Input: part model. Units: mm. Frame: model coordinates. Face numbers are marked on the shaded views. Coordinates: 2 decimals unless noted, no trailing zeros. Order: outer loops, then holes, each group sorted by start corner. A loop starts at its lowest first (then second) coordinate and runs counter-clockwise, first axis right, second up. Notation, with made-up numbers: (24.25, 63) - (73.25, 63) arc R32 cw to (73.25, 99) - close; hole circle Ø7 at (41, -28.5). An arc over 180 degrees is marked (long way). Answer as CSV lines item,"result". Start each with the question number.
Item 1: Material intervals for line 1 along Y through (x, z) = (20, -2.8); line 2 along X through (y, z) = (-1.25, -0.8); line 3 along X through (y, z) = (-1, -3.4), sorted ascending.
Item 2: Section A-A (y = 0). Output: boundary loops of the cut face in (x, z), and give its area (4 significant figures).
Item 3: Section B-B (z = -2.3). Output: boundary loops of the cut face in (x, y).
Item 4: Draft query along Y for the marked faces 1, 2 and 3. Return one class per face: +Y half, -Y half, draft (parallel to the pull), parting line (faces both ways), or undercut.
Item 5: First-contact query: pin 1 (6 mm diameter, centred on x = -20, y = 0, fed in from +Z); pin 2 (1.5 mm diameter, centred on y = 2, z = -2.5, fed in from +X). Flat tips, straight axial feed; report the tip coordinate or a pass-through.
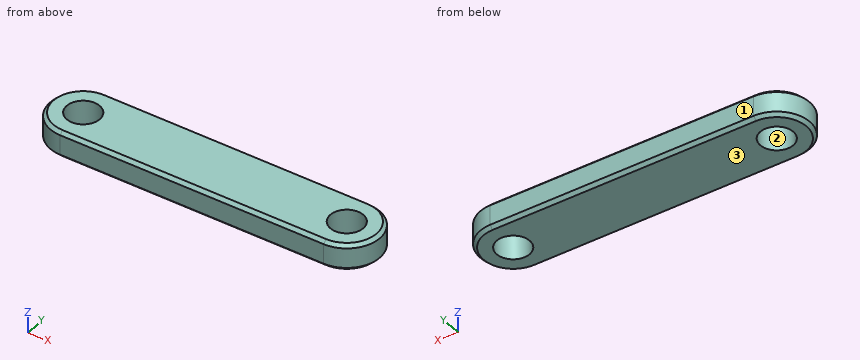
from build123d import *

# Parameters (mm, degrees)
SKETCH1_R           = 2.5
BOSS_EXTRUDE1_DEPTH = 4
CHAMFER1_SIZE       = 0.5


with BuildPart() as part:
    # Sketch1 → Boss-Extrude1 (new body)
    with BuildSketch(Plane.XY):
        with BuildLine():
            Line((-20, 5), (20, 5))
            ThreePointArc((20, 5), (25, 0), (20, -5))
            Line((20, -5), (-20, -5))
            ThreePointArc((-20, -5), (-25, 0), (-20, 5))
        make_face()
        with Locations((-20, 0)):
            Circle(SKETCH1_R, mode=Mode.SUBTRACT)
        with Locations((20, 0)):
            Circle(SKETCH1_R, mode=Mode.SUBTRACT)
    extrude(amount=-BOSS_EXTRUDE1_DEPTH)

    # Chamfer1
    chamfer1_edges = [part.edges().sort_by_distance(p)[0] for p in [
        (25, 0, -4),
        (0, 5, -4),
        (-25, 0, -4),
        (0, 5, 0),
        (25, 0, 0),
        (0, -5, 0),
        (-25, 0, 0),
        (0, -5, -4),
    ]]
    chamfer(chamfer1_edges, length=CHAMFER1_SIZE)


solid = part.part
Determined:
1,line 1,"y = -5 to -2.5, 2.5 to 5"
1,line 2,"x = -24.84 to -22.17, -17.83 to 17.83, 22.17 to 24.84"
1,line 3,"x = -24.9 to -22.29, -17.71 to 17.71, 22.29 to 24.9"
2,outline,"(-25, -3.5) - (-24.5, -4) - (-22.5, -4) - (-22.5, 0) - (-24.5, 0) - (-25, -0.5) - close; (-17.5, -4) - (17.5, -4) - (17.5, 0) - (-17.5, 0) - close; (22.5, -4) - (24.5, -4) - (25, -3.5) - (25, -0.5) - (24.5, 0) - (22.5, 0) - close"
2,area,"159.5 mm^2"
3,outline,"(-20, -5) - (20, -5) arc R5 ccw to (20, 5) - (-20, 5) arc R5 ccw to start; hole circle Ø5 at (-20, 0); hole circle Ø5 at (20, 0)"
4,face 1,"+Y half"
4,face 2,"undercut"
4,face 3,"draft"
5,pin 1,"stops at z = 0"
5,pin 2,"stops at x = 24.84"
